```python
from build123d import *

# Parameters (mm, degrees)
F_01_BASE_PROFILE_W           = 220
F_01_BASE_PROFILE_H           = 48
F_01_BASE_PROFILE_R           = 7.5
F_01_BASE_PROFILE_W_2         = 60
F_01_BASE_PROFILE_H_2         = 15
F_01_BASE_EXTRUDE_DEPTH       = 28
F_02_BOSS_PROFILE_W           = 42
F_02_BOSS_PROFILE_H           = 48
F_02_REINFORCEMENT_BOSS_DEPTH = 42


with BuildPart() as part:
    # 01_Base_Profile → 01_Base_Extrude (new body)
    with BuildSketch(Plane(origin=(0, 0, 0), x_dir=(1, 0, 0), z_dir=(0, 1, 0))):
        Rectangle(F_01_BASE_PROFILE_W, F_01_BASE_PROFILE_H)
        with Locations(Location((-78, 0, 0), (0, 0, 270))):
            Circle(F_01_BASE_PROFILE_R, mode=Mode.SUBTRACT)
        with Locations(Location((-42, 0, 0), (0, 0, 270))):
            Circle(F_01_BASE_PROFILE_R, mode=Mode.SUBTRACT)
        with Locations((45, 0)):
            Rectangle(F_01_BASE_PROFILE_W_2, F_01_BASE_PROFILE_H_2, mode=Mode.SUBTRACT)
    extrude(amount=F_01_BASE_EXTRUDE_DEPTH)

    # 02_Boss_Profile → 02_Reinforcement_Boss (add)
    with BuildSketch(Plane(origin=(0, 0, 0), x_dir=(1, 0, 0), z_dir=(0, 1, 0))):
        with Locations((80, 0)):
            Rectangle(F_02_BOSS_PROFILE_W, F_02_BOSS_PROFILE_H)
    extrude(amount=F_02_REINFORCEMENT_BOSS_DEPTH)


solid = part.part
```
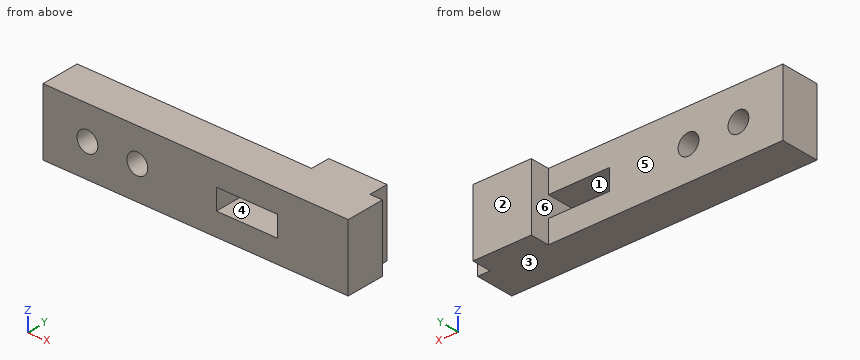
Work out the finished part from the listing and answer in its coordinate system (mm). Face numbers are marked on the shaded views. A direction names the side the tool comes from. Coordinates: 2 decimals unless noted, no trailing zeros. Write each loop counter-clockwise with the first axis right and the second up, starting at its lowest first coordinate (ties: lowest second). Pieces come first, ordered by that corner, then holes.
Q1. Find the intervals of material crossed by line 1 (X direction, y = 10.5, z = 0); line 2 (X direction, y = 16, z = -3); line 3 (Y direction, x = -14.5, z = 8.5), in increasing order.
Q2. Each of these flat-tipped pins is pushed along its axis until it touches: pin 1 Ø1 at (x, z) = (27, 11.5) entering from +Y; pin 2 Ø24 at (x, z) = (-78, 0) entering from -Y; pin 3 Ø7 at (y, z) = (33, 6.5) entering from +X. Where does it stop, or does it pass through?
Q3. Which of the six approach directions +Z, -Z, +X, -X, +Y, -Y give full straight-line access (tool end or side, diameter ignored) to the marked faces 4, 5 and 6?
Q4. A cutting plane is placed at B-B, the plane y = 6.5. Give the vertices of the cut face in (x, z), then the cut area to 3 significant figures.
Q5. Determine the mould class of the marked faces 1, 2 and 3 for opening direction Z: released by +Z, released by -Z, zero draft, split by the parting line, or undercut.
Q6. A cutting plane is placed at A-A, the plane x = 20. Give the vertices of the cut face in (y, z), then the cut area to 3 significant figures.
Q7. A cutting plane is placed at C-C, the plane z = 2.5. Give the vertices of the cut face in (x, y).
Q8. A cutting plane is placed at D-D, the plane z = -19. Give the vertices of the cut face in (x, y), then the cut area to 3 significant figures.
Findings below:
1. line 1: x = -110 to -85.5, -70.5 to -49.5, -34.5 to 15, 59 to 110
1. line 2: x = -110 to -84.87, -71.13 to -48.87, -35.13 to 15, 59 to 110
1. line 3: y = 0 to 28
2. pin 1: stops at y = 28
2. pin 2: stops at y = 0
2. pin 3: stops at x = 101
3. face 4: +Y, -Y
3. face 5: +Z, -Z, -X, +Y
3. face 6: +Y
4. outline: (-110, -24) - (110, -24) - (110, 24) - (-110, 24) - close; hole circle Ø15 at (-78, 0); hole circle Ø15 at (-42, 0); hole (15, -7.5) - (59, -7.5) - (59, 7.5) - (15, 7.5) - close
4. area: 9,550 mm2
5. face 1: undercut
5. face 2: zero draft
5. face 3: released by -Z
6. outline: (0, -24) - (28, -24) - (28, -7.5) - (0, -7.5) - close; (0, 7.5) - (28, 7.5) - (28, 24) - (0, 24) - close
6. area: 924 mm2
7. outline: (-110, 0) - (-85.07, 0) - (-85.07, 28) - (-110, 28) - close; (-70.93, 0) - (-49.07, 0) - (-49.07, 28) - (-70.93, 28) - close; (-34.93, 0) - (15, 0) - (15, 28) - (-34.93, 28) - close; (59, 0) - (110, 0) - (110, 28) - (101, 28) - (101, 42) - (59, 42) - close
8. outline: (-110, 0) - (110, 0) - (110, 28) - (101, 28) - (101, 42) - (59, 42) - (59, 28) - (-110, 28) - close
8. area: 6,750 mm2
